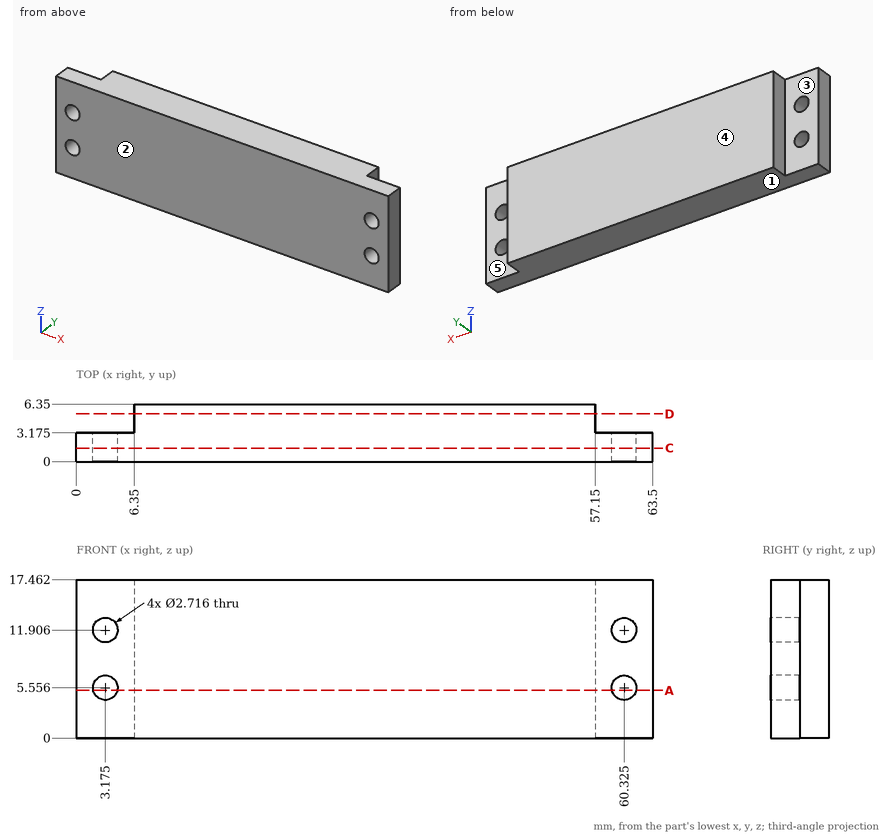
Geometry: see drawing. Coordinates: mm, zero at the bounding-box minimum. A direction names the side the tool comes from. Round coordinates to 2 decimals unless told otherwise and drop trailing zeros. Loops run counter-clockwise (first coordinate to the right, second up) from the corner with the lowest first, then second, coordinate; pieces in that order, holes last. Notation, with made-up numbers: (24.5, 68.25) -> (62.5, 68.25) arc R15 ccw to (62.5, 88.25) -> close; hole circle Ø11 at (36, 19.25). An arc over 180 degrees is marked (long way). Write each question's results on one line, items separated by ' | '.
1. Mould query, pull axis Y, two halves, no side actions, for the marked faces 1, 2 and 3. Classes: +Y half, -Y half, draft (parallel to the pull), parting line (faces both ways), or undercut.
Geometry results:
face 1: draft | face 2: -Y half | face 3: +Y half
2. First-contact query: P1, Ø3.5, axis at x = 60.32, z = 11.91, coming from the -Y side; P2, Ø2, axis at x = 3.17, z = 11.91, coming from the -Y side; P3, Ø3.5, axis at y = 5, z = 13, coming from the +X side; P4, Ø3.5, axis at y = 5.5, z = 9, coming from the -X side. Flat tips, straight axial feed; report the tip coordinate or a pass-through.
Geometry results:
P1: y = 0 | P2: through | P3: x = 57.15 | P4: x = 6.35
3. Set-up query: the marked faces 4 and 5. Return all of +Z, -Z, +X, -X, +Y, -Y with unobstructed straight access to the full face (end or side cutting, diameter ignored); none if empty.
Geometry results:
face 4: +Z, -Z, +X, -X, +Y | face 5: +Z, -Z, +X, +Y
4. Ray query, line 1 (X direction, y = 1, z = 6); line 2 (X direction, y = 5.25, z = 9). Return the intervals inside material, ascending. Write a range as from..to.
Geometry results:
line 1: 0..1.89, 4.46..59.04, 61.61..63.5 | line 2: 6.35..57.15
5. Section A-A (z = 5.25). State how many separate pieces and enclosed holes the cut face has, and give its area (3 significant figures).
Geometry results:
separate pieces: 3 | enclosed holes: 0 | area: 346 mm2
6. Section C-C (y = 1.5). Return loops of the section in (x, z) (1 decimal), and give its area (3 significant figures).
Geometry results:
outline: (0, 0) -> (63.5, 0) -> (63.5, 17.5) -> (0, 17.5) -> close; hole circle Ø2.7 at (3.2, 5.6); hole circle Ø2.7 at (3.2, 11.9); hole circle Ø2.7 at (60.3, 5.6); hole circle Ø2.7 at (60.3, 11.9) | area: 1,090 mm2
7. Section D-D (y = 5.25). Return loops of the section in (x, z).
Geometry results:
outline: (6.35, 0) -> (57.15, 0) -> (57.15, 17.46) -> (6.35, 17.46) -> close
